Geometry check sheet. Reference: the model listing, model coordinates, mm. A direction names the side the tool comes from. Give positions to 0.01 mm unless a question says otherwise; leave off trailing zeros. Loops run counter-clockwise (first coordinate to the right, second up) from the corner with the lowest first, then second, coordinate; pieces in that order, holes last.
Autodesk Inventor part; units mm, degrees
ref_plane "YZ Plane" through (0, 0, 0) normal (1, 0, 0) x (0, 1, 0)
ref_plane "XZ Plane" through (0, 0, 0) normal (0, 1, 0) x (-1, 0, 0)
ref_plane "XY Plane" through (0, 0, 0) normal (0, 0, 1) x (1, 0, 0)
sketch "Sketch1" plane through (0, 0, 0) normal (0, 0, 1) x (1, 0, 0)
  line L0 (5.5, 2.5) -> (5.5, 12)
  line L1 (5.5, 12) -> (3.5, 12)
  line L2 (3.5, 12) -> (3.5, 9.93)
  line L3 (3.5, 9.93) -> (0, 9.93)
  line L4 (5.5, 2.5) -> (0, 2.5)
  line L5 (0, 2.5) -> (0, 9.93)
  line L6 (-2.3, 0) -> (6.8, 0)
  line L7 (0, 0) -> (0, 17.5)
  line L8 (0, 9) -> (0, 2.5)
  line L9 (0, 15) -> (0, 9)
  point P0 (0, 6.215)
  point P1 (-1, 12)
  point P2 (4.5, 12)
  dimension "d0" = 5.5
  dimension "d1" = 3.5
  dimension "d2" = 9.93
  dimension "d3" = 12
  dimension "d4" = 2.5
  dimension "d8" = 1
revolve "Revolution1" add sketch "Sketch1" angle 360 about axis through (-10, 0, 0) along (1, 0, 0)
mirror "Mirror2" about plane through (0, 0, 0) normal (1, 0, 0) of "Revolution1"
properties part number "Belt_Pulley" material "Aluminum 6061"
1) Tool access check on faces 1 (the flat face through (5.5, 0, 3)), 2 (the cylindrical face through (0.049, -2.153, -9.694)). Record the directions out of +Z, -Z, +X, -X, +Y, -Y that give a thin tool (end or side, any length) a straight path to the whole face; none if there is none.
2) Scan lines: line 1 along X through (y, z) = (-9, -6.5); line 2 along Z through (x, y) = (-2.25, 0); line 3 along Y through (x, z) = (3, 2.25). Record each from-to range of solid material in increasing order.
3) Depth check by flat-ended pin: P1, Ø1, axis at x = 3.5, z = 4.5, coming from the +Y side; P2, Ø3, axis at x = -1.5, y = -7, coming from the +Z side; P3, Ø3, axis at x = 3, z = 8.5, coming from the -Y side. Enter the tip coordinate at first touch or a pass-through.
4) Sectioned sample at A-A on z = 0. Enter the section's corners in (x, y).
5) Sectioned sample at D-D on z = -9. Enter the section's corners in (x, y), plus the area to 3 significant figures.
6) Mould release check, pull along X, two halves, no side actions. Record for faces 3 (the flat face through (-5.5, 0, 3)), 4 (the flat face through (3.5, -5, 9)), 5 (the cylindrical face through (-4.49, -11.99, 0.53)): +X half, -X half, draft (parallel to the pull), parting line (faces both ways), or undercut.
7) Sectioned sample at C-C on x = 4.5. Enter the section's corners in (y, z).
Determined:
1. face 1: +Z, -Z, +X, +Y, -Y
1. face 2: none
2. line 1: x = -5.5 to -3.5, 3.5 to 5.5
2. line 2: z = -9.93 to -2.5, 2.5 to 9.93
2. line 3: y = -9.67 to -1.09, 1.09 to 9.67
3. P1: stops at y = 11.31
3. P2: stops at z = 8.27
3. P3: stops at y = -9.68
4. outline: (-5.5, -12) - (-3.5, -12) - (-3.5, -9.93) - (3.5, -9.93) - (3.5, -12) - (5.5, -12) - (5.5, -2.5) - (-5.5, -2.5) - close; (-5.5, 2.5) - (5.5, 2.5) - (5.5, 12) - (3.5, 12) - (3.5, 9.93) - (-3.5, 9.93) - (-3.5, 12) - (-5.5, 12) - close
5. outline: (-5.5, -7.94) - (-3.5, -7.94) - (-3.5, -4.2) - (3.5, -4.2) - (3.5, -7.94) - (5.5, -7.94) - (5.5, 7.94) - (3.5, 7.94) - (3.5, 4.2) - (-3.5, 4.2) - (-3.5, 7.94) - (-5.5, 7.94) - close
5. area: 122 mm2
6. face 3: -X half
6. face 4: undercut
6. face 5: draft
7. outline: circle Ø24 at (0, 0); hole circle Ø5 at (0, 0)
